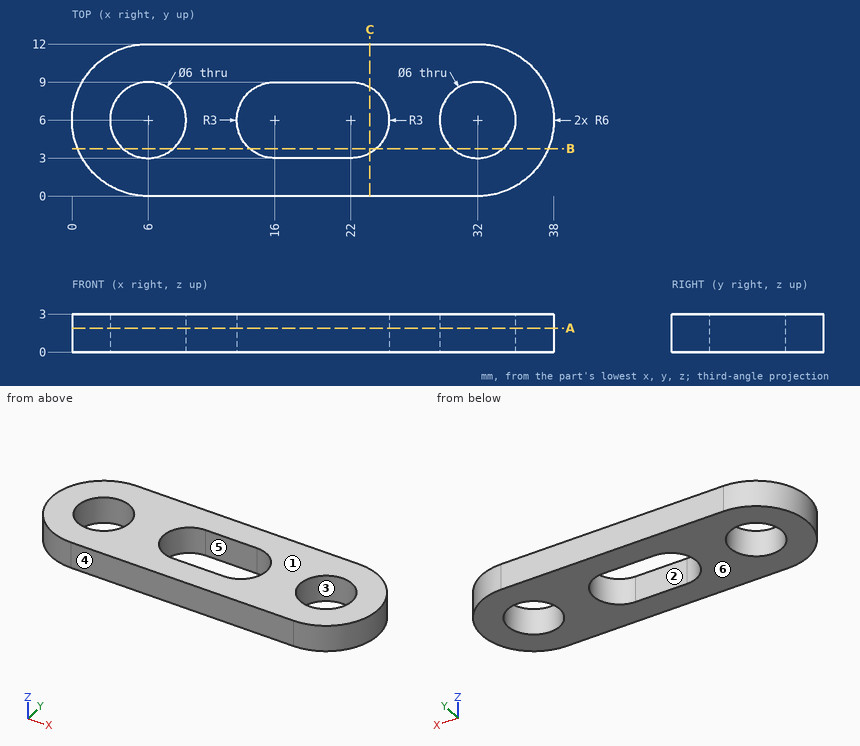
Part print with two shaded views. Sizes in mm from the minimum x, y, z corner. A direction names the side the tool comes from. Round coordinates to 2 decimals unless told otherwise and drop trailing zeros. Write each loop counter-clockwise with the first axis right and the second up, starting at its lowest first coordinate (ties: lowest second). Pieces come first, ordered by that corner, then holes. Notation, with made-up numbers: M 62,78.5 L 82,78.5 A37 cw 82,115.5 Z; hole C 18.25,-24 d1. An arc over 180 degrees is marked long. Answer as CSV lines item,"result". Start each with the question number.
1) Band-saw the part on B-B (y = 3.75). List the corners of the cut face in (x, z).
2) Band-saw the part on C-C (x = 23.5). List the corners of the cut face in (y, z), then the cut area to 3 significant figures.
3) Which spindle directions (+Z, -Z, +X, -X, +Y, -Y) get a long thin tool onto all of the face, cutting with end or side? Do the marked faces 5 and 6. Say none if no direction does.
4) Drill centre lines: L1, parallel to Y at x = 6, z = 1.35; L2, parallel to X at y = 4.5, z = 0.65; L3, parallel to X at y = 5.75, z = 2.05. Where is each one in solid material? Low to high.
5) Drop a flat-ended pin along its axis: pin 1 (3.5 mm diameter, centred on x = 6, y = 6, fed in from +Z). Give the stop position or say it passes through.
6) Band-saw the part on A-A (z = 1.9). List the corners of the cut face in (x, y), then the cut area to 3 significant figures.
7) Mould opens along Y. For the marked faces 1, 2, 3 and 4 say: +Y half, -Y half, draft (parallel to the pull), parting line (faces both ways), or undercut.
Worked out:
1,outline,"M 0.44,0 L 4.02,0 L 4.02,3 L 0.44,3 Z; M 7.98,0 L 14.02,0 L 14.02,3 L 7.98,3 Z; M 23.98,0 L 30.02,0 L 30.02,3 L 23.98,3 Z; M 33.98,0 L 37.56,0 L 37.56,3 L 33.98,3 Z"
2,outline,"M 0,0 L 3.4,0 L 3.4,3 L 0,3 Z; M 8.6,0 L 12,0 L 12,3 L 8.6,3 Z"
2,area,"20.4 mm²"
3,face 5,"+Z, -Z"
3,face 6,"-Z, +X, -X, +Y, -Y"
4,L1,"0 to 3, 9 to 12"
4,L2,"0.19 to 3.4, 8.6 to 13.4, 24.6 to 29.4, 34.6 to 37.81"
4,L3,"0.01 to 3.01, 8.99 to 13.01, 24.99 to 29.01, 34.99 to 37.99"
5,pin 1,"through"
6,outline,"M 6,0 L 32,0 A6 ccw 32,12 L 6,12 A6 ccw Z; hole C 6,6 d6; hole M 16,3 L 22,3 A3 ccw 22,9 L 16,9 A3 ccw Z; hole C 32,6 d6"
6,area,"304 mm²"
7,face 1,"draft"
7,face 2,"undercut"
7,face 3,"undercut"
7,face 4,"-Y half"
